```python
from build123d import *

# Parameters (mm, degrees)
SKETCH1_W           = 12
SKETCH1_H           = 23
BOSS_EXTRUDE1_DEPTH = 21
SKETCH2_W           = 31
SKETCH2_H           = 1
BOSS_EXTRUDE2_DEPTH = 12
SKETCH3_R           = 6
BOSS_EXTRUDE3_DEPTH = 4
SKETCH4_W           = 5
SKETCH4_H           = 8
BOSS_EXTRUDE4_DEPTH = 3
SKETCH5_R           = 3.5
BOSS_EXTRUDE5_DEPTH = 6


with BuildPart() as part:
    # Sketch1 → Boss-Extrude1 (new body)
    with BuildSketch(Plane(origin=(0, 0, 0), x_dir=(1, 0, 0), z_dir=(0, 1, 0))):
        Rectangle(SKETCH1_W, SKETCH1_H)
    extrude(amount=BOSS_EXTRUDE1_DEPTH)

    # Sketch2 → Boss-Extrude2 (add)
    with BuildSketch(Plane(origin=(6, 0, 0), x_dir=(0, 0, -1), z_dir=(1, 0, 0))):
        with Locations((0, 15.5)):
            Rectangle(SKETCH2_W, SKETCH2_H)
    extrude(amount=-BOSS_EXTRUDE2_DEPTH)

    # Sketch3 → Boss-Extrude3 (add)
    with BuildSketch(Plane(origin=(0, 21, 0), x_dir=(1, 0, 0), z_dir=(0, 1, 0))):
        with Locations(Location((0, -5.5, 0), (0, 0, 270))):
            Circle(SKETCH3_R)
    extrude(amount=BOSS_EXTRUDE3_DEPTH)

    # Sketch4 → Boss-Extrude4 (add)
    with BuildSketch(Plane(origin=(0, 21, 0), x_dir=(1, 0, 0), z_dir=(0, 1, 0))):
        with Locations((0, -1.5)):
            Rectangle(SKETCH4_W, SKETCH4_H)
    extrude(amount=BOSS_EXTRUDE4_DEPTH)

    # Sketch5 → Boss-Extrude5 (add)
    with BuildSketch(Plane(origin=(0, 25, 0), x_dir=(1, 0, 0), z_dir=(0, 1, 0))):
        with Locations(Location((0, -5.5, 0), (0, 0, 270))):
            Circle(SKETCH5_R)
    extrude(amount=BOSS_EXTRUDE5_DEPTH)


solid = part.part
```
The model under review builds one solid part; all positions refer to its coordinate system, in mm. A direction names the side the tool comes from. Give positions to 0.01 mm unless a question says otherwise; leave off trailing zeros. Write each loop counter-clockwise with the first axis right and the second up, starting at its lowest first coordinate (ties: lowest second). Pieces come first, ordered by that corner, then holes. Notation, with made-up numbers: M 58,25.25 L 65,25.25 A21 ccw 65,61.25 Z; hole C 25.5,86 d5. An arc over 180 degrees is marked long. Answer in a Markdown table with one row per item.
Item 1: Add section C-C on z = 13. Give the boundary of the cut face in (x, y), plus the area to 3 significant figures.
Check sheet entries:
| item | result |
|---|---|
| outline | M -6,15 L 6,15 L 6,16 L -6,16 Z |
| area | 12.0 mm2 |
Item 2: Tool access review of faces 1 (the face through (0, 22, -2.5)), 2 (the face through (1.802, 22.972, 11.223)), 3 (the face through (0, 15, 14)): name each direction out of +Z, -Z, +X, -X, +Y, -Y from which nothing blocks a thin tool from reaching the whole face with its end or side.
Check sheet entries:
| item | result |
|---|---|
| face 1 | -Z, +X, -X, +Y |
| face 2 | +Y |
| face 3 | +Z, +X, -X, -Y |
Item 3: For P1, Ø1.3, axis at y = 22, z = -1, coming from the -X side; P2, Ø0.8, axis at y = 22, z = -1.5, coming from the +X side; P3, Ø2, axis at x = -1.5, z = 14, coming from the +Y side, all flat-tipped, find the tip position at first contact; note any pin that passes through.
Check sheet entries:
| item | result |
|---|---|
| P1 | x = -2.5 |
| P2 | x = 2.5 |
| P3 | y = 16 |
Item 4: For line 1 along Z through (x, y) = (-0.25, 9); line 2 along Y through (x, z) = (-0.5, -10); line 3 along Y through (x, z) = (2.5, -14), list the stretches that pass through material, from the lowest coordinate up.
Check sheet entries:
| item | result |
|---|---|
| line 1 | -11.5 to 11.5 |
| line 2 | 0 to 21 |
| line 3 | 15 to 16 |
Item 5: Add section D-D on x = -1.25. Give the boundary of the cut face in (y, z), plus the area to 3 significant figures.
Check sheet entries:
| item | result |
|---|---|
| outline | M 0,-11.5 L 15,-11.5 L 15,-15.5 L 16,-15.5 L 16,-11.5 L 21,-11.5 L 21,-2.5 L 24,-2.5 L 24,-0.37 L 25,-0.37 L 25,2.23 L 31,2.23 L 31,8.77 L 25,8.77 L 25,11.37 L 21,11.37 L 21,11.5 L 16,11.5 L 16,15.5 L 15,15.5 L 15,11.5 L 0,11.5 Z |
| area | 584 mm2 |
Item 6: Add section A-A on x = -4. Give the boundary of the cut face in (y, z).
Check sheet entries:
| item | result |
|---|---|
| outline | M 0,-11.5 L 15,-11.5 L 15,-15.5 L 16,-15.5 L 16,-11.5 L 21,-11.5 L 21,1.03 L 25,1.03 L 25,9.97 L 21,9.97 L 21,11.5 L 16,11.5 L 16,15.5 L 15,15.5 L 15,11.5 L 0,11.5 Z |
Item 7: Add section B-B on y = 23. Give the boundary of the cut face in (x, z).
Check sheet entries:
| item | result |
|---|---|
| outline | M -2.5,-2.5 L 2.5,-2.5 L 2.5,0.05 A6 ccw long -2.5,0.05 Z |
